Design review of the part built by this model. Coordinates are the model's own, in mm. Face numbers are marked on the shaded views. A direction names the side the tool comes from. Round coordinates to 2 decimals unless told otherwise and drop trailing zeros. Loops run counter-clockwise (first coordinate to the right, second up) from the corner with the lowest first, then second, coordinate; pieces in that order, holes last. Notation, with made-up numbers: (-13, 15.25) - (28, 15.25) arc R32 cw to (28, 44.25) - close; hole circle Ø11 at (18, 7). An arc over 180 degrees is marked (long way). Return JSON: item names as keys, results as strings. Group by question number.
(1) For the marked faces 1 and 2, list the 3-axis set-ups (+Z, -Z, +X, -X, +Y, -Y) from which the entire face can be reached by the end or side of a thin tool; tool diameter is ignored.
(2) Clearance check with flat-ended pins moving along their axes: pin 1 (2 mm diameter, centred on x = 25, y = 44, fed in from +Z) (3 decimals); pin 2 (2.5 mm diameter, centred on x = -23.5, z = 35, fed in from +Y); pin 3 (12 mm diameter, centred on y = -21, z = 18.5, fed in from -X); pin 4 (1.6 mm diameter, centred on x = -22.5, z = 25.5, fed in from -Y). State where each tip first meets the part, or that it passes through.
(3) We need section C-C, the plane z = 22.5. Write out the cut boundary in (x, y), and give its area (3 significant figures).
(4) Wall thickness on L1, parallel to Z at x = -15, y = 23 (3 decimals); L2, parallel to X at y = -45, z = 39.5: over which ranges is each line inside the solid? List them lowest first. Write a range as [from, to].
(5) We need section A-A, the plane z = 64.5. Write out the cut boundary in (x, y).
(6) We need section D-D, the plane x = 44.5. Write out the cut boundary in (y, z) (3 decimals).
(7) We need section B-B, the plane y = -28.5. Write out the cut boundary in (x, z) (3 decimals), and give its area (3 significant figures).
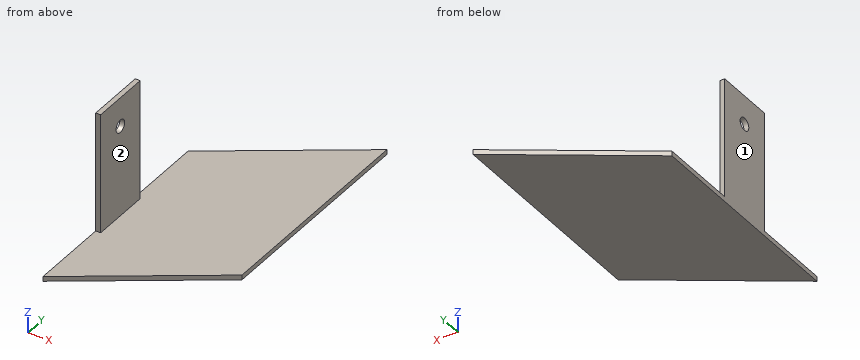
Autodesk Inventor part; units mm, degrees
ref_plane "YZ Plane" through (0, 0, 0) normal (1, 0, 0) x (0, 1, 0)
ref_plane "XZ Plane" through (0, 0, 0) normal (0, 1, 0) x (-1, 0, 0)
ref_plane "XY Plane" through (0, 0, 0) normal (0, 0, 1) x (1, 0, 0)
sketch "Sketch1" plane through (0, 0, 0) normal (0, 0, 1) x (1, 0, 0)
  line L0 (-24.3533, 25.6313) -> (-24.3533, -114.0687)
  line L1 (-24.3533, -114.0687) -> (64.0742, -52.1511)
  line L2 (-24.3533, -114.0687) -> (83.5967, -114.0687) construction
  line L3 (64.0742, -52.1511) -> (64.0742, 87.5489)
  line L4 (64.0742, 87.5489) -> (-24.3533, 25.6313)
  point P0 (0, 0)
  dimension "d0" = 139.7
  dimension "d1" = 107.95
  dimension "d2" = 35
  dimension "d3" = 139.7
extrude "Extrusion1" add sketch "Sketch1" along normal blind 3.175
sketch "Sketch2" plane through (0, 0, 3.175) normal (0, 0, 1) x (1, 0, 0)
  line L0 (-24.3533, 25.6313) -> (-24.3533, -114.0687)
  line L1 (-21.1783, -44.2187) -> (-21.1783, -25.1687)
  line L2 (-21.1783, -25.1687) -> (-24.3533, -25.1687)
  line L3 (-21.1783, -44.2187) -> (-21.1783, -63.2687)
  line L4 (-21.1783, -63.2687) -> (-24.3533, -63.2687)
  line L5 (-24.3533, -25.1687) -> (-24.3533, -63.2687)
  point P0 (0, 0)
  dimension "d7" = 19.05
  dimension "d8" = 19.05
extrude "Extrusion2" add sketch "Sketch2" along normal blind 79.2734
sketch "Sketch3" plane through (-24.3533, -114.0687, 0) normal (-1, 0, 0) x (0, 0, 1)
  line L0 (82.4484, 88.9) -> (63.3984, 88.9)
  line L1 (63.3984, 88.9) -> (63.3984, 69.85)
  line L2 (63.3984, 69.85) -> (82.4484, 69.85)
  line L3 (82.4484, 69.85) -> (82.4484, 88.9)
  point P0 (0, 114.0687)
  dimension "d11" = 19.05
  dimension "d12" = 19.05
hole "Hole1" at (-24.3533, -44.2187, 63.3984) direction (1, 0, 0) diameter 8.3312 end through all
properties part number "Right Abdomen"
Solutions:
{
 "1": {"face 1": "+Z, -Z, -X, +Y, -Y", "face 2": "+Z, +X, +Y, -Y"},
 "2": {"pin 1": "z = 3.175", "pin 2": "y = -25.17", "pin 3": "x = -24.35", "pin 4": "y = -63.27"},
 "3": {"outline": "(-24.35, -63.27) - (-21.18, -63.27) - (-21.18, -25.17) - (-24.35, -25.17) - close", "area": "121 mm^2"},
 "4": {"L1": "[0, 3.175]", "L2": "[-24.35, -21.18]"},
 "5": {"outline": "(-24.35, -63.27) - (-21.18, -63.27) - (-21.18, -48.24) - (-24.35, -48.24) - close; (-24.35, -40.2) - (-21.18, -40.2) - (-21.18, -25.17) - (-24.35, -25.17) - close"},
 "6": {"outline": "(-65.857, 0) - (73.843, 0) - (73.843, 3.175) - (-65.857, 3.175) - close"},
 "7": {"outline": "(-24.353, 0) - (64.074, 0) - (64.074, 3.175) - (-21.178, 3.175) - (-21.178, 82.448) - (-24.353, 82.448) - close", "area": "532 mm^2"}
}
